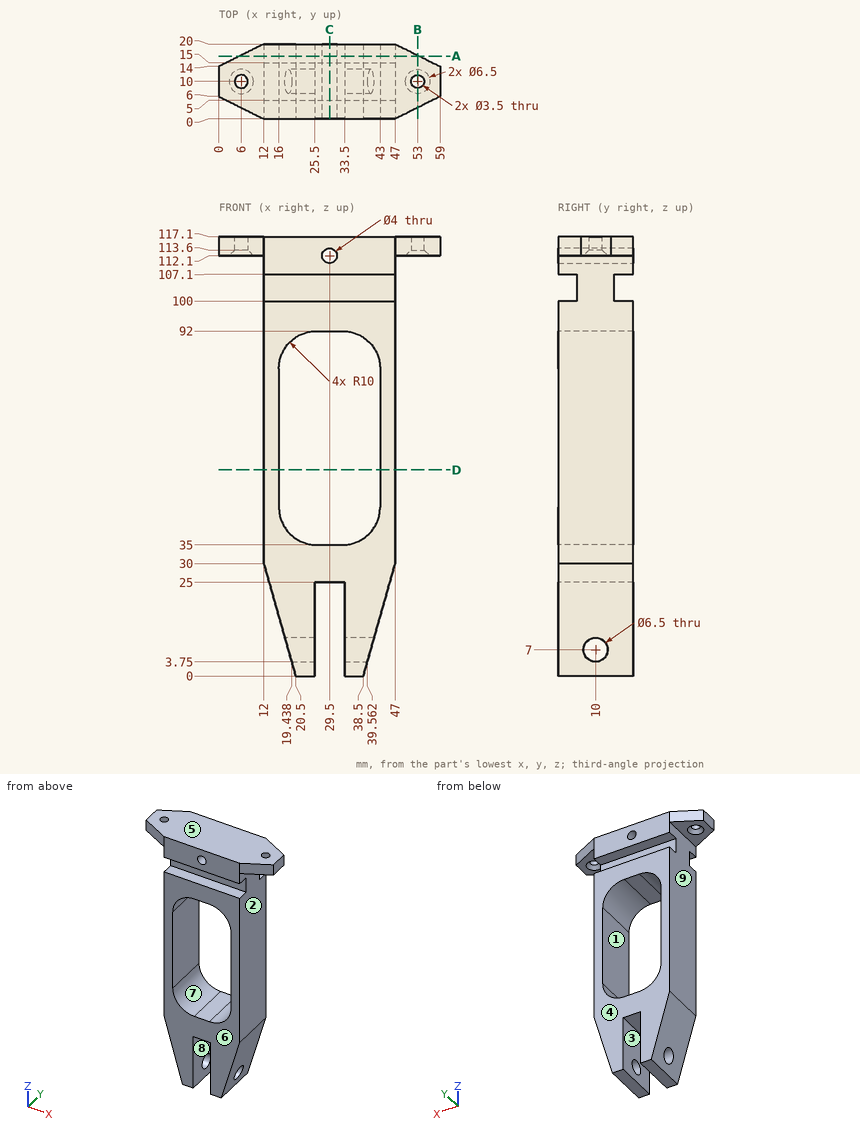
Input: dimensioned drawing with shaded views. Units: mm. Origin: part minimum x, y, z. A direction names the side the tool comes from. Coordinates: 2 decimals unless noted, no trailing zeros. Write each loop counter-clockwise with the first axis right and the second up, starting at its lowest first coordinate (ties: lowest second). Pieces come first, ordered by that corner, then holes. Notation, with made-up numbers: M 89,47 L 121,47 A22 cw 121,72 Z; hole C -10,33.25 d10. An arc over 180 degrees is marked long. Use one line per item in the form item = value.
Q1. Section C-C (x = 29.5). Return loops of the section in (y, z), plus the area to 3 significant figures.
Answer below:
outline = M 0,25 L 20,25 L 20,35 L 0,35 Z; M 0,92 L 20,92 L 20,100 L 15,100 L 15,107.1 L 20,107.1 L 20,110.1 L 0,110.1 L 0,107.1 L 5,107.1 L 5,100 L 0,100 Z; M 0,114.1 L 20,114.1 L 20,117.1 L 0,117.1 Z
area = 551 mm²
Q2. Draft query along X for the marked faces 6, 7, 8 and 9. Return one class per face: released by +X, released by -X, zero draft, split by the parting line, or undercut.
Answer below:
face_6 = zero draft
face_7 = undercut
face_8 = undercut
face_9 = released by -X
Q3. Set-up query: the marked faces 1, 2, 3, 4 and 5. Return all of +Z, -Z, +X, -X, +Y, -Y with unobstructed straight access to the full face (end or side cutting, diameter ignored); none if empty.
Answer below:
face_1 = +Y, -Y
face_2 = -Z, +X, +Y, -Y
face_3 = -Z, +Y, -Y
face_4 = +Z, -Z, +X, -X, +Y
face_5 = +Z, +X, -X, +Y, -Y
Q4. Section D-D (z = 55). Return loops of the section in (x, y).
Answer below:
outline = M 12,0 L 16,0 L 16,20 L 12,20 Z; M 43,0 L 47,0 L 47,20 L 43,20 Z
Q5. Section A-A (y = 16.75). Return loops of the section in (x, z).
Answer below:
outline = M 5.5,112.1 L 12,112.1 L 12,107.1 L 47,107.1 L 47,112.1 L 53.5,112.1 L 53.5,117.1 L 5.5,117.1 Z; M 12,30 L 20.5,0 L 25.5,0 L 25.5,25 L 33.5,25 L 33.5,0 L 38.5,0 L 47,30 L 47,100 L 12,100 Z; hole M 16,45 A10 ccw 26,35 L 33,35 A10 ccw 43,45 L 43,82 A10 ccw 33,92 L 26,92 A10 ccw 16,82 Z; hole C 29.5,112.1 d4
Q6. First-contact query: pin 1 (4 mm diameter, centred on x = 28.5, y = 7, fed in from -Z); pin 2 (1 mm diameter, centred on y = 16.5, z = 56, fed in from +X); pin 3 (2 mm diameter, centred on x = 32.5, z = 105, fed in from -Y); pin 4 (3 mm diameter, centred on x = 6, y = 10, fed in from -Z). Flat tips, straight axial feed; report the tip coordinate or a pass-through.
Answer below:
pin_1 = 25
pin_2 = 47
pin_3 = 5
pin_4 = through
Q7. Material intervals for probe 1 along Y at (x, z) = (19, 7); probe 2 along X at (y, z) = (14.25, 58); probe 3 along Z at (x, y) = (26.5, 8.75), sorted ascending. Write a range as from..to.
Answer below:
probe_1 = 0..6.75, 13.25..20
probe_2 = 12..16, 43..47
probe_3 = 25..35, 92..117.1
Q8. Section B-B (x = 53). Return loops of the section in (y, z).
Answer below:
outline = M 3,112.1 L 6.75,112.1 L 8.25,113.6 L 8.25,117.1 L 3,117.1 Z; M 11.75,113.6 L 13.25,112.1 L 17,112.1 L 17,117.1 L 11.75,117.1 Z
